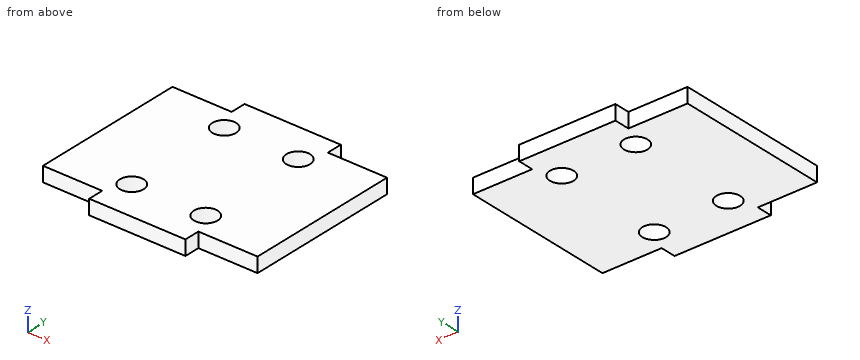
from build123d import *

# Parameters (mm, degrees)
SKETCH_1_W      = 29
SKETCH_1_H      = 21
SKETCH_1_R      = 1.6
SKETCH_1_W_2    = 13
SKETCH_1_H_2    = 2.1
EXTRUDE_1_DEPTH = 2


with BuildPart() as part:
    # 草图1 → 凸台-拉伸1 (new body)
    # profile 1 of 3: a face of its own
    with BuildSketch(Plane.XY):
        with Locations((14.5, 10.5)):
            Rectangle(SKETCH_1_W, SKETCH_1_H)
        with Locations((9.5, 18)):
            Circle(SKETCH_1_R, mode=Mode.SUBTRACT)
        with Locations((19.5, 18)):
            Circle(SKETCH_1_R, mode=Mode.SUBTRACT)
        with Locations((9.5, 3)):
            Circle(SKETCH_1_R, mode=Mode.SUBTRACT)
        with Locations((19.5, 3)):
            Circle(SKETCH_1_R, mode=Mode.SUBTRACT)
    # profile 2 of 3: a face of its own
    with BuildSketch(Plane.XY):
        with Locations((14.5, -1.05)):
            Rectangle(SKETCH_1_W_2, SKETCH_1_H_2)
    # profile 3 of 3: a face of its own
    with BuildSketch(Plane.XY):
        with Locations((14.5, 22.05)):
            Rectangle(SKETCH_1_W_2, SKETCH_1_H_2)
    extrude(amount=EXTRUDE_1_DEPTH)


solid = part.part
Read the model definition and answer for the solid it produces. Units are mm, in the model's axes. Coordinates: 2 decimals unless noted, no trailing zeros. Loops run counter-clockwise (first coordinate to the right, second up) from the corner with the lowest first, then second, coordinate; pieces in that order, holes last. Notation, with made-up numbers: (39.25, 57.5) -> (47.25, 57.5) arc R22 cw to (47.25, 81.5) -> close; hole circle Ø9 at (21, -26). An arc over 180 degrees is marked (long way). Write item = value, one per line. Start each with the question number.
1) Find the intervals of material crossed by L1, parallel to Y at x = 9.5, z = 1.5; L2, parallel to X at y = 17.25, z = 0.8; L3, parallel to X at y = 3.25, z = 1.3, in increasing order. Write a range as from..to.
2) Given P1, Ø1, axis at y = 9.5, z = 0.5, coming from the -X side; P2, Ø1, axis at y = 22.5, z = 1.5, coming from the -X side; P3, Ø1, axis at x = 24, z = 1, coming from the -Y side; P4, Ø1.9, axis at x = 9.5, y = 18, coming from the +Z side, each flat-ended and moving along its own axis, determine where each tip first touches the part or whether it passes through.
3) The part is cut by section A-A, the plane z = 1. Determine the outline of the cut face in (x, y), plus the area to 3 significant figures.
4) The part is cut by section B-B, the plane x = 19.5. Determine the outline of the cut face in (y, z).
5) The part is cut by section D-D, the plane x = 5. Determine the outline of the cut face in (y, z), plus the area to 3 significant figures.
6) The part is cut by section C-C, the plane y = 3. Determine the outline of the cut face in (x, z), plus the area to 3 significant figures.
Result:
q1.L1 = -2.1..1.4, 4.6..16.4, 19.6..23.1
q1.L2 = 0..8.09, 10.91..18.09, 20.91..29
q1.L3 = 0..7.92, 11.08..17.92, 21.08..29
q2.P1 = 0
q2.P2 = 8
q2.P3 = 0
q2.P4 = through
q3.outline = (0, 0) -> (8, 0) -> (8, -2.1) -> (21, -2.1) -> (21, 0) -> (29, 0) -> (29, 21) -> (21, 21) -> (21, 23.1) -> (8, 23.1) -> (8, 21) -> (0, 21) -> close; hole circle Ø3.2 at (9.5, 3); hole circle Ø3.2 at (9.5, 18); hole circle Ø3.2 at (19.5, 3); hole circle Ø3.2 at (19.5, 18)
q3.area = 631 mm²
q4.outline = (-2.1, 0) -> (1.4, 0) -> (1.4, 2) -> (-2.1, 2) -> close; (4.6, 0) -> (16.4, 0) -> (16.4, 2) -> (4.6, 2) -> close; (19.6, 0) -> (23.1, 0) -> (23.1, 2) -> (19.6, 2) -> close
q5.outline = (0, 0) -> (21, 0) -> (21, 2) -> (0, 2) -> close
q5.area = 42.0 mm²
q6.outline = (0, 0) -> (7.9, 0) -> (7.9, 2) -> (0, 2) -> close; (11.1, 0) -> (17.9, 0) -> (17.9, 2) -> (11.1, 2) -> close; (21.1, 0) -> (29, 0) -> (29, 2) -> (21.1, 2) -> close
q6.area = 45.2 mm²
